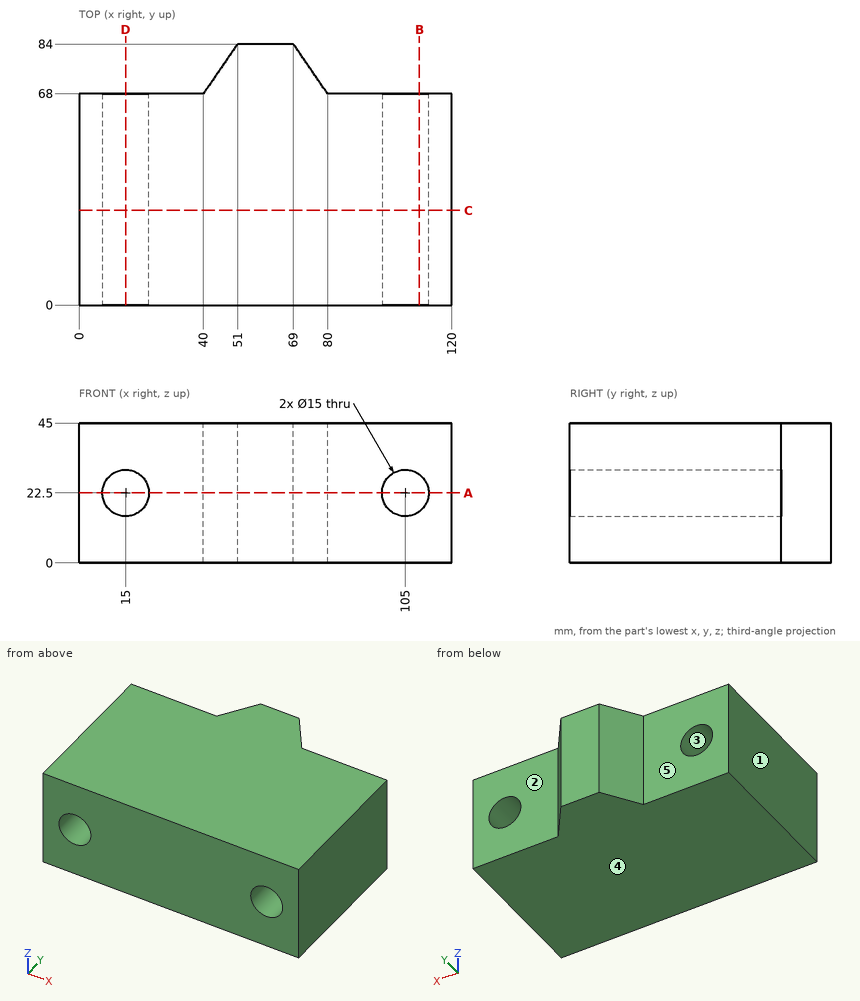
Verification items for this drawing (mm, ordinates from the low corner). A direction names the side the tool comes from. Give positions to 0.01 mm unless a question says otherwise; leave off trailing zeros. Loops run counter-clockwise (first coordinate to the right, second up) from the corner with the lowest first, then second, coordinate; pieces in that order, holes last. Notation, with made-up numbers: M 83.5,24.5 L 93.5,24.5 A20 ccw 93.5,58.5 Z; hole C 79,61 d1. An arc over 180 degrees is marked long. Write item = value, one per line. Start each with the question number.
1. Section check D-D, the plane x = 15. Enter the section's corners in (y, z).
2. Section check B-B, the plane x = 109.5. Enter the section's corners in (y, z).
3. Thickness scan on probe 1 along X at (y, z) = (30, 23); probe 2 along Z at (x, y) = (15, 40.5); probe 3 along X at (y, z) = (7, 24.5). Record the ranges inside material, lowest first.
4. Draft check along X on the marked faces 1, 2 and 3. Enter one of: +X half, -X half, draft (parallel to the pull), parting line (faces both ways), or undercut.
5. Section check A-A, the plane z = 22.5. Enter the section's corners in (x, y).
6. Go/stop test with flat-tipped pins: P1, Ø6, axis at x = 49.5, y = 52.5, coming from the -Z side; P2, Ø20, axis at x = 15.5, z = 29.5, coming from the +Y side; P3, Ø9, axis at x = 105, z = 22.5, coming from the +Y side. Record where each tip stops, or that it passes through.
7. Tool access check on the marked faces 4 and 5. Record the directions out of +Z, -Z, +X, -X, +Y, -Y that give a thin tool (end or side, any length) a straight path to the whole face; none if there is none.
8. Section check C-C, the plane y = 30.5. Enter the section's corners in (x, z).
Values follow:
q1.outline = M 0,0 L 68,0 L 68,15 L 0,15 Z; M 0,30 L 68,30 L 68,45 L 0,45 Z
q2.outline = M 0,0 L 68,0 L 68,16.5 L 0,16.5 Z; M 0,28.5 L 68,28.5 L 68,45 L 0,45 Z
q3.probe_1 = 0 to 7.52, 22.48 to 97.52, 112.48 to 120
q3.probe_2 = 0 to 15, 30 to 45
q3.probe_3 = 0 to 7.77, 22.23 to 97.77, 112.23 to 120
q4.face_1 = -X half
q4.face_2 = draft
q4.face_3 = undercut
q5.outline = M 0,0 L 7.5,0 L 7.5,68 L 0,68 Z; M 22.5,0 L 97.5,0 L 97.5,68 L 80,68 L 69,84 L 51,84 L 40,68 L 22.5,68 Z; M 112.5,0 L 120,0 L 120,68 L 112.5,68 Z
q6.P1 = 0
q6.P2 = 68
q6.P3 = through
q7.face_4 = -Z, +X, -X, +Y, -Y
q7.face_5 = +Z, -Z, -X, +Y
q8.outline = M 0,0 L 120,0 L 120,45 L 0,45 Z; hole C 15,22.5 d15; hole C 105,22.5 d15
